```python
from build123d import *

# Parameters (mm, degrees)
EXTRUDE_1_DEPTH     = 9
CUT_EXTRUDE_START   = -5
CUT_EXTRUDE_1_DEPTH = 5
SKETCH_12_W         = 2.5
SKETCH_12_H         = 7
CUT_EXTRUDE_3_DEPTH = 42.911887352
FILLET_11_R         = 2
FILLET_1_R          = 1
SKETCH_10_W         = 8
SKETCH_10_H         = 4
EXTRUDE_3_DEPTH     = 2
FILLET_5_R          = 5
FILLET_10_R         = 7.5
FILLET_14_R         = 2
FILLET_15_R         = 1.5
FILLET_16_R         = 2
FILLET_17_R         = 1
FILLET_18_R         = 2
SKETCH_11_R         = 5.6
CUT_EXTRUDE_2_DEPTH = 44.514365603


# Some blends are built 0.0001 mm under size
with BuildPart() as part:
    # Эскиз2 → Бобышка-Вытянуть1 (new body)
    with BuildSketch(Plane.XY):
        with BuildLine():
            Line((-18, 0), (-15, 0))
            Line((-15, 0), (-15, 7))
            Line((-15, 7), (-10, 7))
            Line((-10, 7), (-10, 0))
            ThreePointArc((-10, 0), (-7.39984978, -6.726233956), (-0.951555354, -9.954624172))
            ThreePointArc((-0.951555354, -9.954624172), (10.407523967, -15.498539394), (15.320888862, -27.144247806))
            ThreePointArc((15.320888862, -27.144247806), (8.452365235, -21.873844259), (0, -20))
            ThreePointArc((0, -20), (-1.44344914, -20.176216472), (-2.802111775, -20.69451514))
            ThreePointArc((-2.802111775, -20.69451514), (-7.346697493, -22.426064476), (-12.174852362, -23.009539415))
            ThreePointArc((-12.174852362, -23.009539415), (-16.488233618, -23.738589268), (-20.315570084, -25.857142338))
            ThreePointArc((-20.315570084, -25.857142338), (-31.05163084, -24.430323259), (-29.168151763, -13.764896883))
            ThreePointArc((-29.168151763, -13.764896883), (-22.544234788, -7.726123715), (-18, 0))
        make_face()
    extrude(amount=EXTRUDE_1_DEPTH)

    # Эскиз6 → Вырез-Вытянуть1 (cut)
    with BuildSketch(Plane.XY.offset(9).offset(CUT_EXTRUDE_START)):
        with BuildLine():
            ThreePointArc((-9.55, -2.96605799), (-16.390256677, -12.316180922), (-16.898984287, -23.890078556))
            ThreePointArc((-16.898984287, -23.890078556), (-14.577958647, -23.229625817), (-12.174852362, -23.009539415))
            ThreePointArc((-12.174852362, -23.009539415), (-7.346697493, -22.426064476), (-2.802111775, -20.69451514))
            ThreePointArc((-2.802111775, -20.69451514), (-1.44344914, -20.176216472), (0, -20))
            ThreePointArc((0, -20), (8.452365235, -21.873844259), (15.320888862, -27.144247806))
            ThreePointArc((15.320888862, -27.144247806), (10.407523967, -15.498539394), (-0.951555354, -9.954624172))
            ThreePointArc((-0.951555354, -9.954624172), (-6.307192762, -7.760110789), (-9.55, -2.96605799))
        make_face()
    extrude(amount=CUT_EXTRUDE_1_DEPTH, mode=Mode.SUBTRACT)

    # Эскиз12 → Вырез-Вытянуть3 (cut, through all)
    with BuildSketch(Plane.ZY.offset(15)):
        with Locations((1.25, 3.5)):
            Rectangle(SKETCH_12_W, SKETCH_12_H)
        with Locations((7.75, 3.5)):
            Rectangle(SKETCH_12_W, SKETCH_12_H)
    extrude(amount=-CUT_EXTRUDE_3_DEPTH, mode=Mode.SUBTRACT)

    # Скругление11
    fillet_11_edges = [part.edges().sort_by_distance(p)[0] for p in [
        (-10, 0, 7.75),
        (-10, 0, 1.25),
    ]]
    fillet(fillet_11_edges, radius=FILLET_11_R)

    # Скругление1
    fillet_1_edges = [part.edges().sort_by_distance(p)[0] for p in [
        (15.320888862, -27.144247806, 2),
    ]]
    fillet(fillet_1_edges, radius=FILLET_1_R)

    # Эскиз10 → Бобышка-Вытянуть3 (add)
    with BuildSketch(Plane(origin=(0, 7, 0), x_dir=(-1, 0, 0), z_dir=(0, 1, 0))):
        with Locations((14, 4.5)):
            Rectangle(SKETCH_10_W, SKETCH_10_H)
    extrude(amount=EXTRUDE_3_DEPTH)

    # Скругление5
    fillet_5_edges = [part.edges().sort_by_distance(p)[0] for p in [
        (-10, 9, 4.5),
    ]]
    fillet(fillet_5_edges, radius=FILLET_5_R)

    # Скругление10
    fillet_10_edges = [part.edges().sort_by_distance(p)[0] for p in [
        (-16.898984287, -23.890078556, 6.5),
    ]]
    fillet(fillet_10_edges, radius=FILLET_10_R - 0.0001)  # a hair under: the kernel refuses the full size

    # Скругление14
    fillet_14_edges = [part.edges().sort_by_distance(p)[0] for p in [
        (-15, 7, 4.5),
    ]]
    fillet(fillet_14_edges, radius=FILLET_14_R)

    # Скругление15
    fillet_15_edges = [part.edges().sort_by_distance(p)[0] for p in [
        (-17.5, 7, 6.5),
        (-15, 2.5, 6.5),
        (-17.5, 7, 2.5),
        (-15.585786438, 6.414213562, 2.5),
        (-15.585786438, 6.414213562, 6.5),
        (-15, 2.5, 2.5),
    ]]
    fillet(fillet_15_edges, radius=FILLET_15_R)

    # Скругление16
    # the kernel refuses this fillet: 2 mm, written as the material it adds along each edge
    with BuildSketch(Plane(origin=(-11.832159566, -2, 6.5), x_dir=(-0.6907726827654878, -0.7230719886325089, 0), z_dir=(-0.7230719886325089, 0.6907726827654878, 0))) as fillet_16_piece_1_section:
        with BuildLine():
            CenterArc((2 + FILLET_16_R, FILLET_16_R), FILLET_16_R, 180, 90)
            Line((2, FILLET_16_R), (2, 0))
            Line((2, 0), (2 + FILLET_16_R, 0))
        make_face()
    fillet_16_piece_1 = revolve(axis=Axis((-11.832159566, -2, 6.5), (0, 0, 1)), revolution_arc=223.691304566, mode=Mode.PRIVATE)
    fillet_16_piece_1 = split(fillet_16_piece_1, bisect_by=Plane(origin=(-9.962064569, 0, 7.231915875), z_dir=(0, -1, 0)), keep=Keep.TOP, mode=Mode.PRIVATE)
    fillet_16_piece_1 = fillet_16_piece_1 - Plane(origin=(0, 0, 7.231915875), x_dir=(-1, 0, 0), z_dir=(0, 0, -1)) * Cylinder(10, 17, mode=Mode.PRIVATE)
    fillet_16_piece_1 = fillet_16_piece_1 - Plane(origin=(2.479707116, -18.943734501, 7.231915875), x_dir=(-0.6014853558135568, 0.7988838255602869, 0), z_dir=(0, 0, -1)) * Cylinder(20, 17, mode=Mode.PRIVATE)
    add(fillet_16_piece_1)
    with BuildSketch(Plane(origin=(-11.832159566, -2, 6.5), x_dir=(-0.6907726827654878, -0.7230719886325089, 0), z_dir=(-0.7230719886325089, 0.6907726827654878, 0))) as fillet_16_piece_2_section:
        with BuildLine():
            CenterArc((2 + FILLET_16_R, FILLET_16_R), FILLET_16_R, 180, 90)
            Line((2, FILLET_16_R), (2, 0))
            Line((2, 0), (2 + FILLET_16_R, 0))
        make_face()
    fillet_16_piece_2 = revolve(axis=Axis((-11.832159566, -2, 6.5), (0, 0, 1)), revolution_arc=223.691304566, mode=Mode.PRIVATE)
    fillet_16_piece_2 = split(fillet_16_piece_2, bisect_by=Plane(origin=(-11.088968436, 0, 6.841402023), z_dir=(0, 1, 0)), keep=Keep.TOP, mode=Mode.PRIVATE)
    fillet_16_piece_2 = split(fillet_16_piece_2, bisect_by=Plane(origin=(-10, 0.441530369, 6.841402023), z_dir=(-1, 0, 0)), keep=Keep.TOP, mode=Mode.PRIVATE)
    add(fillet_16_piece_2)
    with BuildSketch(Plane(origin=(-13.5, 0, 6.5), x_dir=(0, 0, 1), z_dir=(1, 0, 0))) as fillet_16_piece_3:
        with BuildLine():
            CenterArc((FILLET_16_R, -FILLET_16_R), FILLET_16_R, 90, 90)
            Line((0, -FILLET_16_R), (0, 0))
            Line((0, 0), (FILLET_16_R, 0))
        make_face()
    extrude(amount=1.667840434)
    with BuildSketch(Plane(origin=(-11.832159566, -2, 2.5), x_dir=(-0.6907726827654875, -0.7230719886325091, 0), z_dir=(-0.7230719886325091, 0.6907726827654875, 0))) as fillet_16_piece_4_section:
        with BuildLine():
            CenterArc((2 + FILLET_16_R, -FILLET_16_R), FILLET_16_R, 90, 90)
            Line((2, -FILLET_16_R), (2, 0))
            Line((2, 0), (2 + FILLET_16_R, 0))
        make_face()
    fillet_16_piece_4 = revolve(axis=Axis((-11.832159566, -2, 2.5), (0, 0, 1)), revolution_arc=223.691304566, mode=Mode.PRIVATE)
    fillet_16_piece_4 = split(fillet_16_piece_4, bisect_by=Plane(origin=(-9.962064569, 0, 1.768084125), z_dir=(0, -1, 0)), keep=Keep.TOP, mode=Mode.PRIVATE)
    fillet_16_piece_4 = fillet_16_piece_4 - Plane(origin=(0, 0, 1.768084125), x_dir=(-1, 0, 0), z_dir=(0, 0, -1)) * Cylinder(10, 17, mode=Mode.PRIVATE)
    add(fillet_16_piece_4)
    with BuildSketch(Plane(origin=(-11.832159566, -2, 2.5), x_dir=(-0.6907726827654875, -0.7230719886325091, 0), z_dir=(-0.7230719886325091, 0.6907726827654875, 0))) as fillet_16_piece_5_section:
        with BuildLine():
            CenterArc((2 + FILLET_16_R, -FILLET_16_R), FILLET_16_R, 90, 90)
            Line((2, -FILLET_16_R), (2, 0))
            Line((2, 0), (2 + FILLET_16_R, 0))
        make_face()
    fillet_16_piece_5 = revolve(axis=Axis((-11.832159566, -2, 2.5), (0, 0, 1)), revolution_arc=223.691304566, mode=Mode.PRIVATE)
    fillet_16_piece_5 = split(fillet_16_piece_5, bisect_by=Plane(origin=(-10, 0.441530341, 2.15859789), z_dir=(-1, 0, 0)), keep=Keep.TOP, mode=Mode.PRIVATE)
    add(fillet_16_piece_5)
    with BuildSketch(Plane(origin=(-13.5, 0, 2.5), x_dir=(0, 0, -1), z_dir=(1, 0, 0))) as fillet_16_piece_6:
        with BuildLine():
            CenterArc((FILLET_16_R, FILLET_16_R), FILLET_16_R, 180, 90)
            Line((0, FILLET_16_R), (0, 0))
            Line((0, 0), (FILLET_16_R, 0))
        make_face()
    extrude(amount=1.667840434)
    with BuildSketch(Plane(origin=(-13.5, 0, 4), x_dir=(0, 0, -1), z_dir=(1, 0, 0))) as fillet_16_piece_7:
        with BuildLine():
            CenterArc((1.5 + FILLET_16_R, FILLET_16_R), FILLET_16_R, 180, 90)
            Line((1.5 + FILLET_16_R, 0), (1.5, 0))
            Line((1.5, 0), (1.5, FILLET_16_R))
        make_face()
    revolve(axis=Axis((-13.5, 0, 4), (0, 1, 0)), revolution_arc=90)
    with BuildSketch(Plane(origin=(-15, 0, 4), x_dir=(0, 1, 0), z_dir=(0, 0, 1))) as fillet_16_piece_8:
        with BuildLine():
            CenterArc((FILLET_16_R, FILLET_16_R), FILLET_16_R, 180, 90)
            Line((0, FILLET_16_R), (0, 0))
            Line((0, 0), (FILLET_16_R, 0))
        make_face()
    extrude(amount=1)
    with BuildSketch(Plane(origin=(-13.5, 0, 5), x_dir=(0, 0, 1), z_dir=(1, 0, 0))) as fillet_16_piece_9:
        with BuildLine():
            CenterArc((1.5 + FILLET_16_R, -FILLET_16_R), FILLET_16_R, 90, 90)
            Line((1.5 + FILLET_16_R, 0), (1.5, 0))
            Line((1.5, 0), (1.5, -FILLET_16_R))
        make_face()
    revolve(axis=Axis((-13.5, 0, 5), (0, -1, 0)), revolution_arc=90)

    # Скругление17
    fillet_17_edges = [part.edges().sort_by_distance(p)[0] for p in [
        (-18, 8.75, 2.5),
        (-18, 7.439339828, 2.939339828),
        (-18, 7, 4.5),
        (-18, 8.75, 6.5),
        (-18, 7.439339828, 6.060660172),
    ]]
    fillet(fillet_17_edges, radius=FILLET_17_R - 0.0001)  # a hair under: the kernel refuses the full size

    # Скругление18
    fillet_18_edges = [part.edges().sort_by_distance(p)[0] for p in [
        (-9.55, -2.96605799, 5.25),
    ]]
    fillet(fillet_18_edges, radius=FILLET_18_R)

    # Эскиз11 → Вырез-Вытянуть2 (cut, through all)
    with BuildSketch(Plane.XY.offset(9)):
        with Locations((-25, -20)):
            Circle(SKETCH_11_R)
    extrude(amount=-CUT_EXTRUDE_2_DEPTH, mode=Mode.SUBTRACT)


solid = part.part
```
Read the model definition and answer for the solid it produces. Units are mm, in the model's axes. A direction names the side the tool comes from. Give positions to 0.01 mm unless a question says otherwise; leave off trailing zeros. Order: outer loops, then holes, each group sorted by start corner. A loop starts at its lowest first (then second) coordinate and runs counter-clockwise, first axis right, second up. Notation, with made-up numbers: (-24.75, 6.25) -> (26.25, 6.25) arc R36 cw to (26.25, 42.25) -> close; hole circle Ø3 at (4, -37). An arc over 180 degrees is marked (long way). One line per item, written item: value. Start each with the question number.
(1) Straight lines are drawn through the part: L1, parallel to X at y = -25, z = 1.25; L2, parallel to Y at x = -25, z = 6; L3, parallel to Z at x = -2.5, y = -12. For each, find the intervals that lie inside material, in ascending order.
(2) A tool of negligible diameter and unlimited length cuts with its end or side. For faces 5 (the flat face through (-20, -14, 9)), 6 (the cylindrical face through (-10.556, -0.46, 8.753)), 7 (the cylindrical face through (-17.699, 8.754, 2.785)), 8 (the flat face through (-3, -16, 4)), 9 (the cylindrical face through (7.207, -21.343, 1.972)), from which of +Z, -Z, +X, -X, +Y, -Y can it reach the whole face along a straight path? Write none if from no direction.
(3) Flat-ended cylindrical pins translate along their axes: P1, Ø0.5, axis at y = 8.5, z = 5, coming from the -X side; P2, Ø1, axis at x = -0.5, z = 5.5, coming from the -Y side; P3, Ø3, axis at y = 1.5, z = 5, coming from the +X side; P4, Ø5.5, axis at x = -14.5, y = 5, coming from the -Z side. Find the tip coordinate at first contact, or state that the pin passes through.
(4) The part is cut by section A-A (x = -27.5). Determine the outline of the cut face in (y, z).
(5) The part is cut by section C-C (x = -3.5). Determine the outline of the cut face in (y, z), and give its area (3 significant figures).
(6) For a pull along Y with two mould halves and no side action, classify faces 1 (the cylindrical face through (9.186, -14.324, 1.972)), 2 (the cylindrical face through (-14.55, 3.52, 2.93)), 3 (the flat face through (-13, 5, 2.5)), 4 (the cylindrical face through (-15.6, 0.57, 4.49)) as released by +Y, released by -Y, zero draft, split by the parting line, or undercut.
(7) The part is cut by section B-B (x = 11.5). Determine the outline of the cut face in (y, z), and give its area (3 significant figures).
Taken from the geometry:
1. L1: -30.59 to -27.52, -22.48 to -19.11, 13.23 to 14.68
1. L2: -27.5 to -25.6, -14.4 to -10.4
1. L3: 0 to 4
2. face 5: +Z, +X, -X, +Y, -Y
2. face 6: +Z, +X, +Y
2. face 7: -Z, -X, +Y
2. face 8: +Z, +X, -Y
2. face 9: +Z, -Z, -Y
3. P1: x = -18
3. P2: through
3. P3: x = -10
3. P4: z = 2.5
4. outline: (-27.07, 0) -> (-25.01, 0) -> (-25.01, 9) -> (-27.07, 9) -> close; (-14.99, 0) -> (-12.57, 0) -> (-12.57, 9) -> (-14.99, 9) -> close
5. outline: (-21.05, 0) -> (-9.37, 0) -> (-9.37, 4) -> (-21.05, 4) -> close
5. area: 46.7 mm^2
6. face 1: released by +Y
6. face 2: undercut
6. face 3: zero draft
6. face 4: undercut
7. outline: (-23.64, 0) -> (-16.77, 0) -> (-16.77, 4) -> (-23.64, 4) -> close
7. area: 27.5 mm^2
